Autodesk Fusion 360 part; units mm, degrees
box "BoxPrimitive1" add length 10 width 6 height 15 placed x (0, 1, 0) y (0, 0, 1) z (1, 0, 0) at (0, 0, 0)
sketch "Sketch3" plane through (0, 0, 0) normal (-1, 0, 0) x (0, 0, 1)
  line L0 (6, 10) -> (0, 10)
  line L1 (0, 10) -> (0, 0)
  line L2 (0, 0) -> (6, 0)
  line L3 (6, 0) -> (6, 10)
  line L4 (3, 10) -> (3, 6.5) construction
  line L5 (4.75, 10) -> (1.25, 10)
  line L6 (1.25, 10) -> (1.25, 3)
  line L7 (1.25, 3) -> (4.75, 3)
  line L8 (4.75, 3) -> (4.75, 10)
  line L9 (4.75, 10) -> (1.25, 3) construction
  line L10 (1.25, 10) -> (4.75, 3) construction
  point P0 (3, 6.5)
  dimension "d11" = 3.5
  dimension "d12" = 3.5
  dimension "d13" = 7
extrude "Extrude1" cut sketch "Sketch3" against normal blind 15 contours L0 L5 L6 L7 L8
equation "Hole = 3.5 mm"
equation "Width = 6 mm"
equation "Length = 15 mm"
equation "d4 = Height"
equation "d5 = Width"
equation "d6 = Length"
equation "Height = 10 mm"
equation "HHole = 7 mm"
equation "d11 = HHole / 2"
equation "d12 = Hole"
equation "d13 = HHole"
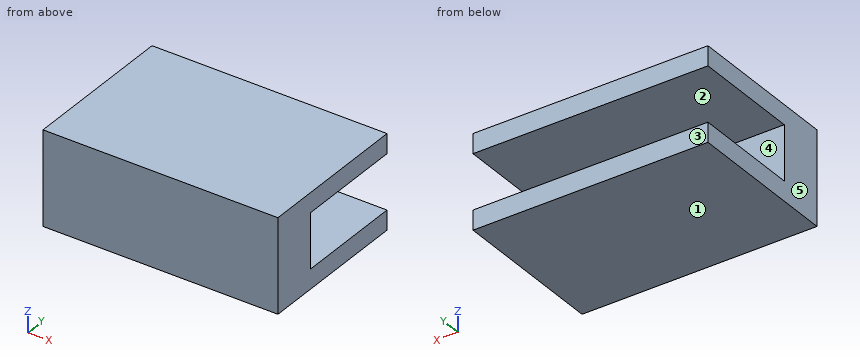
CAD build for the part. Positions are in the model's coordinates, mm. Face numbers are marked on the shaded views. A direction names the side the tool comes from. Coordinates: 2 decimals unless noted, no trailing zeros. Write each loop counter-clockwise with the first axis right and the second up, starting at its lowest first coordinate (ties: lowest second). Pieces come first, ordered by that corner, then holes. Notation, with made-up numbers: (-3.5, -30.5) -> (3.5, -30.5) arc R28 ccw to (3.5, 5.5) -> close; hole circle Ø9 at (72, 22). An arc over 180 degrees is marked (long way). Use CSV: the item, a comma, the result in double quotes. Start each with the question number.
Item 1: Band-saw the part on C-C, the plane z = 2.85. Write the cut outline in (x, y).
Item 2: Two-plate mould, pull along Z, no slides. Class the marked faces 1, 2 and 3: +Z half, -Z half, draft (parallel to the pull), parting line (faces both ways), or undercut.
Item 3: Band-saw the part on B-B, the plane x = 3.25. Write the cut outline in (y, z).
Item 4: Band-saw the part on A-A, the plane y = 4. Write the cut outline in (x, z), plus the area to 3 significant figures.
Item 5: Drop a flat-ended pin along its axis: P1, Ø1.8, axis at x = 8, z = 3, coming from the +Y side. Give the stop position or say it passes through.
Item 6: Wall check: probe 1 along Z at (x, y) = (8.25, 4); probe 2 along Y at (x, z) = (13.25, 2.75). Give the ranges that are in metal, low to high.
Item 7: Tool access for the marked faces 4 and 5: list every direction of +Z, -Z, +X, -X, +Y, -Y with a clear straight run to the whole face (end or side of a thin tool).
Response values:
1,outline,"(0, 0) -> (15, 0) -> (15, 3) -> (0, 3) -> close"
2,face 1,"-Z half"
2,face 2,"undercut"
2,face 3,"draft"
3,outline,"(0, 0) -> (10, 0) -> (10, 1.25) -> (3, 1.25) -> (3, 4.75) -> (10, 4.75) -> (10, 6) -> (0, 6) -> close"
4,outline,"(0, 0) -> (15, 0) -> (15, 1.25) -> (0, 1.25) -> close; (0, 4.75) -> (15, 4.75) -> (15, 6) -> (0, 6) -> close"
4,area,"37.5 mm2"
5,P1,"stops at y = 3"
6,probe 1,"z = 0 to 1.25, 4.75 to 6"
6,probe 2,"y = 0 to 3"
7,face 4,"+X, -X, +Y"
7,face 5,"+Z, -Z, -X, +Y, -Y"
